```python
from build123d import *

# Parameters (mm, degrees)
SKETCH1_W           = 15
SKETCH1_H           = 18.3
SKETCH1_W_2         = 44.4
SKETCH1_R           = 2.6
BOSS_EXTRUDE1_DEPTH = 2
SKETCH1_3_W         = 15
SKETCH1_3_H         = 18.3
BOSS_EXTRUDE2_DEPTH = 17
SKETCH2_R           = 6.5
CUT_EXTRUDE2_DEPTH  = 12.315
FILLET3_SIZE        = 4
FILLET4_SIZE        = 3
CHAMFER2_SIZE       = 1


with BuildPart() as part:
    # Sketch1 → Boss-Extrude1 (new body)
    # profile 1 of 3: a face of its own
    with BuildSketch(Plane(origin=(0, 0, 0), x_dir=(1, 0, 0), z_dir=(0, 1, 0))):
        with Locations((-7.5, 9.15)):
            Rectangle(SKETCH1_W, SKETCH1_H)
    # profile 2 of 3: a face of its own
    with BuildSketch(Plane(origin=(0, 0, 0), x_dir=(1, 0, 0), z_dir=(0, 1, 0))):
        with Locations((22.2, 9.15)):
            Rectangle(SKETCH1_W_2, SKETCH1_H)
        with Locations(Location((32.2, 9.15, 0), (0, 0, 270))):
            Circle(SKETCH1_R, mode=Mode.SUBTRACT)
        with Locations(Location((12.2, 9.15, 0), (0, 0, 270))):
            Circle(SKETCH1_R, mode=Mode.SUBTRACT)
    # profile 3 of 3: a face of its own
    with BuildSketch(Plane(origin=(0, 0, 0), x_dir=(1, 0, 0), z_dir=(0, 1, 0))):
        with Locations((51.9, 9.15)):
            Rectangle(SKETCH1_W, SKETCH1_H)
    extrude(amount=BOSS_EXTRUDE1_DEPTH)

    # Sketch1<3> → Boss-Extrude2 (add)
    with BuildSketch(Plane(origin=(0, 0, 0), x_dir=(1, 0, 0), z_dir=(0, 1, 0))):
        with Locations((51.9, 9.15)):
            Rectangle(SKETCH1_3_W, SKETCH1_3_H)
        with Locations((-7.5, 9.15)):
            Rectangle(SKETCH1_3_W, SKETCH1_3_H)
    extrude(amount=BOSS_EXTRUDE2_DEPTH)

    # Sketch2 → Cut-Extrude2 (cut)
    with BuildSketch(Plane.XY):
        with Locations((-7.5, 9.5)):
            Circle(SKETCH2_R)
        with Locations((51.9, 9.5)):
            Circle(SKETCH2_R)
    extrude(amount=-CUT_EXTRUDE2_DEPTH, mode=Mode.SUBTRACT)

    # Fillet3
    fillet3_edges = [part.edges().sort_by_distance(p)[0] for p in [
        (59.4, 0, -9.15),
        (-15, 0, -9.15),
        (44.4, 17, -9.15),
        (59.4, 17, -9.15),
        (-15, 17, -9.15),
        (0, 17, -9.15),
    ]]
    chamfer(fillet3_edges, length=FILLET3_SIZE)

    # Fillet4
    fillet4_edges = [part.edges().sort_by_distance(p)[0] for p in [
        (44.4, 2, -9.15),
        (0, 2, -9.15),
    ]]
    chamfer(fillet4_edges, length=FILLET4_SIZE)

    # Chamfer2
    chamfer2_edges = [part.edges().sort_by_distance(p)[0] for p in [
        (22.2, 0, -18.3),
        (22.2, 0, 0),
    ]]
    chamfer(chamfer2_edges, length=CHAMFER2_SIZE)


solid = part.part
```
Model file for the job. Use its own axes, mm. A direction names the side the tool comes from. Coordinates: 2 decimals unless noted, no trailing zeros. Write each loop counter-clockwise with the first axis right and the second up, starting at its lowest first coordinate (ties: lowest second). Pieces come first, ordered by that corner, then holes. Notation, with made-up numbers: (48, -9) - (88, -9) arc R32 cw to (88, 28) - close; hole circle Ø11 at (23, 48). An arc over 180 degrees is marked (long way). Use a Markdown table: item, result. Add a question column.
Item 1: Two-plate mould, pull along X, no slides. Class faces 1 (the face through (21.7, 1.8, -18.3)), 2 (the face through (57.4, 2, -9)), 3 (the face through (22, 2, -9)): pulls with the +X half, pulls with the -X half, needs draft (parallel to the pull), parting line crosses it, or undercut.
Item 2: Band-saw the part on A-A, the plane y = 9.5. Write the cut outline in (x, z) (3 decimals), and give its area (3 significant figures).
Item 3: Band-saw the part on D-D, the plane z = -5.5. Write the cut outline in (x, y), and give its area (3 significant figures).
Item 4: Drop flat-ended pins along their axis: pin 1 (5 mm diameter, centred on x = 16.5, y = 3, fed in from +Z); pin 2 (1 mm diameter, centred on y = 2, z = -2, fed in from -X); pin 3 (1.5 mm diameter, centred on y = 14, z = -4, fed in from +X); pin 4 (6.5 mm diameter, centred on x = -5.5, y = 10.5, fed in from +Z) (3 decimals). Give the stop position or say it passes through.
Item 5: Band-saw the part on C-C, the plane z = -8.25. Write the cut outline in (x, y).
Item 6: 3-axis set-ups, long thin cutter, end or side, ignore diameter. For faces 4 (the face through (-1.3, 11.45, -6.07)), 5 (the face through (-2, 15, -9)), 6 (the face through (-13, 2, -9)): which of +Z, -Z, +X, -X, +Y, -Y reach the whole face in a straight line?
Item 7: Drill centre lines: line 1 along X through (y, z) = (9.75, -7); line 2 along X through (y, z) = (14.75, -4); line 3 along X through (y, z) = (14, -14.25). Where is each one in solid material? Low to high.
Item 8: Band-saw the part on B-B, the plane x = 32.2. Write the cut outline in (y, z).
A:
| question | item | result |
|---|---|---|
| 1 | face 1 | needs draft |
| 1 | face 2 | pulls with the +X half |
| 1 | face 3 | undercut |
| 2 | outline | (-15, -18.3) - (0, -18.3) - (0, 0) - (-1, 0) - (-1, -12.315) - (-14, -12.315) - (-14, 0) - (-15, 0) - close; (44.4, -18.3) - (59.4, -18.3) - (59.4, 0) - (58.4, 0) - (58.4, -12.315) - (45.4, -12.315) - (45.4, 0) - (44.4, 0) - close |
| 2 | area | 229 mm² |
| 3 | outline | (-15, 4) - (-11, 0) - (55.4, 0) - (59.4, 4) - (59.4, 13) - (55.4, 17) - (48.4, 17) - (44.4, 13) - (44.4, 5) - (41.4, 2) - (3, 2) - (0, 5) - (0, 13) - (-4, 17) - (-11, 17) - (-15, 13) - close; hole circle Ø13 at (-7.5, 9.5); hole circle Ø13 at (51.9, 9.5) |
| 3 | area | 294 mm² |
| 4 | pin 1 | stops at z = 0 |
| 4 | pin 2 | stops at x = -13.5 |
| 4 | pin 3 | stops at x = 59.15 |
| 4 | pin 4 | stops at z = -12.315 |
| 5 | outline | (-15, 4) - (-11, 0) - (9.76, 0) - (9.76, 2) - (3, 2) - (0, 5) - (0, 13) - (-4, 17) - (-11, 17) - (-15, 13) - close; (14.64, 0) - (29.76, 0) - (29.76, 2) - (14.64, 2) - close; (34.64, 0) - (55.4, 0) - (59.4, 4) - (59.4, 13) - (55.4, 17) - (48.4, 17) - (44.4, 13) - (44.4, 5) - (41.4, 2) - (34.64, 2) - close; hole circle Ø13 at (-7.5, 9.5); hole circle Ø13 at (51.9, 9.5) |
| 6 | face 4 | +Z |
| 6 | face 5 | +Z, -Z, +Y |
| 6 | face 6 | +Z, -Z, -X, -Y |
| 7 | line 1 | x = -15 to -14, -1 to 0, 44.4 to 45.4, 58.4 to 59.4 |
| 7 | line 2 | x = -13.25 to -11.33, -3.67 to -1.75, 46.15 to 48.07, 55.73 to 57.65 |
| 7 | line 3 | x = -14 to -1, 45.4 to 58.4 |
| 8 | outline | (0, -17.3) - (1, -18.3) - (2, -18.3) - (2, -11.75) - (0, -11.75) - close; (0, -6.55) - (2, -6.55) - (2, 0) - (1, 0) - (0, -1) - close |
